Geometry: final body of the model. Coordinates: model frame, mm. A direction names the side the tool comes from. Coordinates: 2 decimals unless noted, no trailing zeros. Write each loop counter-clockwise with the first axis right and the second up, starting at its lowest first coordinate (ties: lowest second). Pieces come first, ordered by that corner, then holes.
from build123d import *
from OCP.BRepFilletAPI import BRepFilletAPI_MakeChamfer

# Parameters (mm, degrees)
BOSS_EXTRU_1_DEPTH             = 6
BOSS_EXTRU_5_DEPTH             = 0.575
BOSS_EXTRU_6_REACH             = 39.159
ESQUISSE4_W                    = 0.275
ESQUISSE4_H                    = 6
BOSS_EXTRU_6_DIRECTION_2_REACH = 39.159
BOSS_EXTRU_7_DEPTH             = 2.5
ESQUISSE6_R                    = 1.25
BOSS_EXTRU_8_DEPTH             = 2.5
CHANFREIN1_SIZE                = 1.5
CHANFREIN1_SIZE2               = 0.346302287


with BuildPart() as part:
    # Esquisse1 → Boss.-Extru.1 (new body)
    with BuildSketch(Plane(origin=(0, 0, 0), x_dir=(1, 0, 0), z_dir=(0, 1, 0))):
        Polygon((5, -10.4), (-5, -10.4), (-12.7, -8.229746559), (-12.7, 0.770253441), (-4.765, 14.663984942), (-4.765, 17.6), (4.765, 17.6), (4.765, 14.663984942), (12.7, 0.770253441), (12.7, -8.229746559), align=None)
    extrude(amount=BOSS_EXTRU_1_DEPTH)

    # Esquisse2 → Révolution1 (revolve)
    with BuildSketch(Plane(origin=(0, 0, 0), x_dir=(0, 0, -1), z_dir=(1, 0, 0)), mode=Mode.PRIVATE) as r_volution1_sk:
        Polygon((0, 6), (-9.875, 6), (-9.175, 27.5), (-2.75, 30), (0, 30), align=None)
    revolve(r_volution1_sk.sketch.rotate(Axis((0, 30, 0), (0, -1, 0)), 180), axis=Axis((0, 30, 0), (0, -1, 0)))

    # Esquisse3 → Boss.-Extru.5 (add, symmetric)
    with BuildSketch(Plane(origin=(0, 0, 0), x_dir=(0, 0, -1), z_dir=(1, 0, 0))):
        Polygon((9.175, 27.5), (17.024440931, 24.445742828), (17.875, 6), (9.875, 6), (8.375, 6), (8.375, 27.5), align=None)
    extrude(amount=BOSS_EXTRU_5_DEPTH, both=True)

    # Boss.-Extru.6: up to this face of the body (flat: up to its plane)
    boss_extru_6_end = Plane(part.part.faces().sort_by_distance((4.765, 3, -16.131992471))[0])
    # Esquisse4 → Boss.-Extru.6 (add, up to the picked face)
    with BuildSketch(Plane(origin=(0, 0, 0), x_dir=(0, 0, -1), z_dir=(1, 0, 0)), mode=Mode.PRIVATE) as boss_extru_6_sk1:
        with Locations((17.7375, 3)):
            Rectangle(ESQUISSE4_W, ESQUISSE4_H)
    boss_extru_6_tool1 = split(extrude(boss_extru_6_sk1.sketch, amount=BOSS_EXTRU_6_REACH, mode=Mode.PRIVATE), bisect_by=boss_extru_6_end, keep=Keep.BOTH, mode=Mode.PRIVATE)
    add(boss_extru_6_tool1.solids().sort_by(Axis((0, 3, -17.7375), (1, 0, 0)))[0])

    # Boss.-Extru.6 direction 2: up to this face of the body (flat: up to its plane)
    boss_extru_6_direction_2_end = Plane(part.part.faces().sort_by_distance((-4.765, 3, -16.131992471))[0])
    # Esquisse4 → Boss.-Extru.6 direction 2 (add, up to the picked face)
    with BuildSketch(Plane(origin=(0, 0, 0), x_dir=(0, 0, -1), z_dir=(1, 0, 0)), mode=Mode.PRIVATE) as boss_extru_6_direction_2_sk1:
        with Locations((17.7375, 3)):
            Rectangle(ESQUISSE4_W, ESQUISSE4_H)
    boss_extru_6_direction_2_tool1 = split(extrude(boss_extru_6_direction_2_sk1.sketch, amount=-BOSS_EXTRU_6_DIRECTION_2_REACH, mode=Mode.PRIVATE), bisect_by=boss_extru_6_direction_2_end, keep=Keep.BOTH, mode=Mode.PRIVATE)
    add(boss_extru_6_direction_2_tool1.solids().sort_by(Axis((0, 3, -17.7375), (-1, 0, 0)))[0])

    # Esquisse5 → Boss.-Extru.7 (add, symmetric)
    with BuildSketch(Plane(origin=(0, 0, 0), x_dir=(0, 0, -1), z_dir=(1, 0, 0))):
        Polygon((16.074440931, 24.815392634), (17.024440931, 24.445742828), (17.875, 6), (16.074440931, 6), align=None)
    extrude(amount=BOSS_EXTRU_7_DEPTH, both=True)

    # Esquisse6 → Boss.-Extru.8 (add)
    with BuildSketch(Plane.XZ):
        with Locations(Location((-11, 4.15, 0), (0, 0, 270))):
            Circle(ESQUISSE6_R)
        with Locations(Location((11, 4.15, 0), (0, 0, 90))):
            Circle(ESQUISSE6_R)
    extrude(amount=BOSS_EXTRU_8_DEPTH)

    # Chanfrein1: one chamfer whose edges measure the first distance from different faces: ONE call of the kernel's chamfer builder (chamfer() names one face for all edges)
    chanfrein1_edges_1 = [part.edges().sort_by_distance(p)[0] for p in [
        (-11, -2.5, 5.4),
    ]]
    chanfrein1_side_1 = [part.faces().sort_by_distance(p)[0] for p in [
        (-11, -1.25, 5.4),
    ]]
    chanfrein1_edges_2 = [part.edges().sort_by_distance(p)[0] for p in [
        (11, -2.5, 2.9),
    ]]
    chanfrein1_side_2 = [part.faces().sort_by_distance(p)[0] for p in [
        (11, -1.25, 2.9),
    ]]
    chanfrein1 = BRepFilletAPI_MakeChamfer(part.part.solid().wrapped)
    for e in chanfrein1_edges_1:
        chanfrein1.Add(CHANFREIN1_SIZE, CHANFREIN1_SIZE2, e.wrapped, chanfrein1_side_1[0].wrapped)  # the first distance lies on this face
    for e in chanfrein1_edges_2:
        chanfrein1.Add(CHANFREIN1_SIZE, CHANFREIN1_SIZE2, e.wrapped, chanfrein1_side_2[0].wrapped)  # the first distance lies on this face
    add(Compound.cast(chanfrein1.Shape()), mode=Mode.REPLACE)


solid = part.part
Item 1: Pull-direction query (X, two-part tool) for faces 1 (the flat face through (0.035, 15.352, -17.444)), 2 (the flat face through (8.68, 2.96, -7.81)), 3 (the cylindrical face through (-9.946, -0.493, 3.478)); classes: released by +X, released by -X, zero draft, split by the parting line, or undercut.
Derived:
face 1: zero draft
face 2: released by +X
face 3: undercut
Item 2: Section A-A, the plane y = 5. Output: boundary loops of the cut face in (x, z) (3 decimals), plus the area to 3 significant figures.
Derived:
outline: (-12.7, -0.77) - (-4.765, -14.664) - (-4.765, -17.875) - (4.765, -17.875) - (4.765, -14.664) - (12.7, -0.77) - (12.7, 8.23) - (5, 10.4) - (-5, 10.4) - (-12.7, 8.23) - close
area: 540 mm2
Item 3: Section C-C, the plane y = 20. Output: boundary loops of the cut face in (x, z) (3 decimals), plus the area to 3 significant figures.
Derived:
outline: (-2.5, -17.229) - (2.5, -17.229) - (2.5, -16.074) - (0.575, -16.074) - (0.575, -9.402) arc R9.419 ccw (long way) to (-0.575, -9.402) - (-0.575, -16.074) - (-2.5, -16.074) - close
area: 292 mm2
Item 4: Pin query (flat end, axial travel): pin 1 (0.9 mm diameter, centred on y = 12.5, z = -17, fed in from -X); pin 2 (1 mm diameter, centred on y = 2.5, z = -16.5, fed in from -X) (3 decimals); pin 3 (5 mm diameter, centred on y = 22, z = 2, fed in from +X). Return the tip coordinate at first contact, or that it passes through.
Derived:
pin 1: stops at x = -2.5
pin 2: stops at x = -4.765
pin 3: stops at x = 9.41
Item 5: Section B-B, the plane z = 0. Output: boundary loops of the cut face in (x, y) (3 decimals), plus the area to 3 significant figures.
Derived:
outline: (-12.7, 0) - (12.7, 0) - (12.7, 6) - (9.875, 6) - (9.175, 27.5) - (2.75, 30) - (-2.75, 30) - (-9.175, 27.5) - (-9.875, 6) - (-12.7, 6) - close
area: 592 mm2
Item 6: Section D-D, the plane y = 16.5. Output: boundary loops of the cut face in (x, z) (3 decimals), plus the area to 3 significant figures.
Derived:
outline: (-2.5, -17.391) - (2.5, -17.391) - (2.5, -16.074) - (0.575, -16.074) - (0.575, -9.516) arc R9.533 ccw (long way) to (-0.575, -9.516) - (-0.575, -16.074) - (-2.5, -16.074) - close
area: 300 mm2
Item 7: Material intervals for probe 1 along Y at (x, z) = (9.75, 3.75); probe 2 along X at (y, z) = (21, -13.5) (3 decimals); probe 3 along Y at (x, z) = (-4, 3.5), sorted ascending.
Derived:
probe 1: y = 0 to 6
probe 2: x = -0.575 to 0.575
probe 3: y = 0 to 29
Item 8: Set-up query: faces 4 (the conical face through (0.41, 16.9, 9.51)), 5 (the flat face through (-4.765, 3, -16)), 6 (the flat face through (2.5, 16, -17)). Return all of +Z, -Z, +X, -X, +Y, -Y with unobstructed straight access to the full face (end or side cutting, diameter ignored); none if empty.
Derived:
face 4: +Y
face 5: -Z, -X, +Y, -Y
face 6: -Z, +X, +Y
